CAD build for the part. Positions are in the model's coordinates, mm. A direction names the side the tool comes from. Give positions to 0.01 mm unless a question says otherwise; leave off trailing zeros. Order: outer loops, then holes, each group sorted by start corner. A loop starts at its lowest first (then second) coordinate and runs counter-clockwise, first axis right, second up.
Item 1: Flat gauge pin, fed straight in: P1, Ø1.5, axis at x = -40.5, z = 10, coming from the -Y side. Where does the tip first touch, or does it go through?
Item 2: Band-saw the part on C-C on z = 0. Count the separate pieces of the cut face and the enclosed holes in it, plus the area to 3 significant figures.
Item 3: Two-plate mould, pull along Z, no slides. Class faces 1 (the flat face through (-152.5, -63, 1)), 2 (the flat face through (85, -117, -29)), 3 (the conical face through (-117.265, 7.5, -9.163)): released by +Z, released by -Z, zero draft, split by the parting line, or undercut.
Item 4: Wall check: L1, parallel to X at y = -88, z = 0; L2, parallel to X at y = -126.95, z = 0; L3, parallel to Z at x = 76, y = -27. Give the ranges that are in metal, low to high.
Item 5: Which spindle directions (+Z, -Z, +X, -X, +Y, -Y) get a long thin tool onto all of the face, cutting with end or side? Do faces 4 (the cylindrical face through (46.255, -53.625, 3.905)), 5 (the flat face through (-85, -117, 29)), 6 (the flat face through (-2, 0, -1)). Say none if no direction does.
Item 6: Band-saw the part on B-B on y = -27. Give the cut face in (x, z).
```python
from build123d import *
from OCP.BRepFilletAPI import BRepFilletAPI_MakeChamfer

# Parameters (mm, degrees)
SKETCH1_W           = 305
SKETCH1_H           = 152
BOSS_EXTRUDE1_DEPTH = 127
SKETCH2_R           = 30
CUT_EXTRUDE1_DEPTH  = 213.51176438
BOSS_EXTRUDE2_START = 8
SKETCH3_R           = 45
SKETCH3_R_2         = 30
BOSS_EXTRUDE2_DEPTH = 8
CHAMFER1_SIZE       = 2.911761874
CHAMFER1_SIZE_2     = 8
CUT_EXTRUDE2_START  = -10
SKETCH4_R           = 46
SKETCH4_R_2         = 30
CUT_EXTRUDE2_DEPTH  = 10
CHAMFER2_SIZE       = 3.639702343
CHAMFER2_SIZE_2     = 10
CHAMFER3_SIZE       = 5


with BuildPart() as part:
    # Sketch1 → Boss-Extrude1 (new body)
    with BuildSketch(Plane(origin=(0, 0, 0), x_dir=(1, 0, 0), z_dir=(0, 1, 0))):
        Rectangle(SKETCH1_W, SKETCH1_H)
    extrude(amount=-BOSS_EXTRUDE1_DEPTH)

    # Sketch2 → Cut-Extrude1 (cut, through all)
    with BuildSketch(Plane(origin=(0, 0, 0), x_dir=(1, 0, 0), z_dir=(0, 1, 0))):
        with Locations(Location((-76, 0, 0), (0, 0, 270))):
            Circle(SKETCH2_R)
        with Locations(Location((76, 0, 0), (0, 0, 90))):
            Circle(SKETCH2_R)
    extrude(amount=-CUT_EXTRUDE1_DEPTH, mode=Mode.SUBTRACT)

    # Sketch3 → Boss-Extrude2 (add)
    # profile 1 of 2: a face of its own
    with BuildSketch(Plane(origin=(0, 0, 0), x_dir=(1, 0, 0), z_dir=(0, 1, 0)).offset(BOSS_EXTRUDE2_START)):
        with Locations(Location((-76, 0, 0), (0, 0, 270))):
            Circle(SKETCH3_R)
        with Locations(Location((-76, 0, 0), (0, 0, 270))):
            Circle(SKETCH3_R_2, mode=Mode.SUBTRACT)
    # profile 2 of 2: a face of its own
    with BuildSketch(Plane(origin=(0, 0, 0), x_dir=(1, 0, 0), z_dir=(0, 1, 0)).offset(BOSS_EXTRUDE2_START)):
        with Locations(Location((76, 0, 0), (0, 0, 90))):
            Circle(SKETCH3_R)
        with Locations(Location((76, 0, 0), (0, 0, 90))):
            Circle(SKETCH3_R_2, mode=Mode.SUBTRACT)
    extrude(amount=-BOSS_EXTRUDE2_DEPTH)

    # Chamfer1
    chamfer1_edges_1 = [part.edges().sort_by_distance(p)[0] for p in [
        (-76, 8, -45),
    ]]
    chamfer1_side_1 = [part.faces().sort_by_distance(p)[0] for p in [
        (-76, 8, -44.941764763),
    ]]
    chamfer1_edges_2 = [part.edges().sort_by_distance(p)[0] for p in [
        (76, 8, 45),
    ]]
    chamfer1_side_2 = [part.faces().sort_by_distance(p)[0] for p in [
        (76, 8, 44.941764763),
    ]]
    chamfer1 = BRepFilletAPI_MakeChamfer(part.part.solid().wrapped)
    for e in chamfer1_edges_1:
        chamfer1.Add(CHAMFER1_SIZE - 0.0001, CHAMFER1_SIZE_2 - 0.0001, e.wrapped, chamfer1_side_1[0].wrapped)
    for e in chamfer1_edges_2:
        chamfer1.Add(CHAMFER1_SIZE - 0.0001, CHAMFER1_SIZE_2 - 0.0001, e.wrapped, chamfer1_side_2[0].wrapped)
    add(Compound.cast(chamfer1.Shape()), mode=Mode.REPLACE)  # a hair under: the kernel refuses the full size

    # Sketch4 → Cut-Extrude2 (cut)
    # profile 1 of 2: a face of its own
    with BuildSketch(Plane.XZ.offset(127).offset(CUT_EXTRUDE2_START)):
        with Locations(Location((-76, 0, 0), (0, 0, 270))):
            Circle(SKETCH4_R)
        with Locations(Location((-76, 0, 0), (0, 0, 90))):
            Circle(SKETCH4_R_2, mode=Mode.SUBTRACT)
    # profile 2 of 2: a face of its own
    with BuildSketch(Plane.XZ.offset(127).offset(CUT_EXTRUDE2_START)):
        with Locations(Location((76, 0, 0), (0, 0, 90))):
            Circle(SKETCH4_R)
        with Locations(Location((76, 0, 0), (0, 0, 90))):
            Circle(SKETCH4_R_2, mode=Mode.SUBTRACT)
    extrude(amount=CUT_EXTRUDE2_DEPTH, mode=Mode.SUBTRACT)

    # Chamfer2
    chamfer2_edges_1 = [part.edges().sort_by_distance(p)[0] for p in [
        (-76, -117, 46),
    ]]
    chamfer2_side_1 = [part.faces().sort_by_distance(p)[0] for p in [
        (-76, -117, 45.927205953),
    ]]
    chamfer2_edges_2 = [part.edges().sort_by_distance(p)[0] for p in [
        (76, -117, -46),
    ]]
    chamfer2_side_2 = [part.faces().sort_by_distance(p)[0] for p in [
        (76, -117.072794047, -46),
    ]]
    chamfer2 = BRepFilletAPI_MakeChamfer(part.part.solid().wrapped)
    for e in chamfer2_edges_1:
        chamfer2.Add(CHAMFER2_SIZE - 0.0001, CHAMFER2_SIZE_2 - 0.0001, e.wrapped, chamfer2_side_1[0].wrapped)
    for e in chamfer2_edges_2:
        chamfer2.Add(CHAMFER2_SIZE_2 - 0.0001, CHAMFER2_SIZE - 0.0001, e.wrapped, chamfer2_side_2[0].wrapped)
    add(Compound.cast(chamfer2.Shape()), mode=Mode.REPLACE)  # a hair under: the kernel refuses the full size

    # Chamfer3
    chamfer3_edges = [part.edges().sort_by_distance(p)[0] for p in [
        (0, -127, -76),
        (0, 0, -76),
        (0, 0, 76),
        (-152.5, -63.5, -76),
        (152.5, -63.5, -76),
        (152.5, -63.5, 76),
        (-152.5, -63.5, 76),
        (0, -127, 76),
    ]]
    chamfer(chamfer3_edges, length=CHAMFER3_SIZE)


solid = part.part
```
The answers:
1. P1: stops at y = -117
2. separate pieces: 3
2. enclosed holes: 0
2. area: 23,400 mm2
3. face 1: zero draft
3. face 2: undercut
3. face 3: split by the parting line
4. L1: x = -152.5 to -106, -46 to 46, 106 to 152.5
4. L2: x = -152.5 to -121.98, -30.02 to 30.02, 121.98 to 152.5
4. L3: z = -76 to -30, 30 to 76
5. face 4: +Y, -Y
5. face 5: -Y
5. face 6: +Y
6. outline: (-152.5, -71) - (-147.5, -76) - (147.5, -76) - (152.5, -71) - (152.5, 71) - (147.5, 76) - (-147.5, 76) - (-152.5, 71) - close; hole circle Ø60 at (-76, 0); hole circle Ø60 at (76, 0)
